Autodesk Inventor part; units mm, degrees
ref_plane "YZ Plane" through (0, 0, 0) normal (1, 0, 0) x (0, 1, 0)
ref_plane "XZ Plane" through (0, 0, 0) normal (0, 1, 0) x (-1, 0, 0)
ref_plane "XY Plane" through (0, 0, 0) normal (0, 0, 1) x (1, 0, 0)
sketch "Sketch1" plane through (0, 0, 0) normal (0, 0, 1) x (1, 0, 0)
  line L0 (75, 0) -> (-75, 0)
  line L1 (-75, 0) -> (-75, 150)
  line L2 (-75, 150) -> (75, 150)
  line L3 (75, 150) -> (75, 0)
  point P0 (0, 0)
  point P1 (0, 0)
  dimension "d1" = 150
  dimension "d2" = 150
extrude "Plate1" add sketch "Sketch1" along normal blind 3
sketch "Sketch2" plane through (0, 0, 0) normal (0, 0, 1) x (1, 0, 0)
  line L0 (-75, 0) -> (-75, 150)
  line L1 (75, 0) -> (-75, 0)
  line L2 (75, 150) -> (75, 0)
  line L3 (-75, 150) -> (75, 150)
  circle A0 centre (0, 75) radius 17.5
  line L4 (45, 40) -> (-45, 40) construction
  line L5 (-45, 40) -> (-45, 110) construction
  line L6 (-45, 110) -> (45, 110) construction
  line L7 (45, 110) -> (45, 40) construction
  line L8 (45, 40) -> (-45, 110) construction
  line L9 (-45, 40) -> (45, 110) construction
  circle A1 centre (-45, 40) radius 4
  circle A2 centre (45, 40) radius 4
  circle A3 centre (45, 110) radius 4
  circle A4 centre (-45, 110) radius 4
  point P0 (0, 0)
  point P1 (0, 0)
  point P2 (75, 75)
  dimension "d3" = 35
  dimension "d4" = 90
  dimension "d5" = 70
  dimension "d7" = 8
extrude "Extrusion1" cut sketch "Sketch2" along normal through all contours A1 | A2 | A3 | A4
sketch "Sketch3" plane through (-72, 150, 3) normal (-1, 0, 0) x (0, -1, 0)
  line L0 (150, 0) -> (0, 0)
  line L1 (0, 0) -> (0, -40)
  line L2 (0, -40) -> (150, -40)
  line L3 (150, -40) -> (150, 0)
edge flange "Flange1" height 40 angle 90 thickness 3 bend radius 3 thickness toward (-1, 0, 0) relief tear relief width 3 relief depth 1.5 corner gap 3 corner form 0 edges at (-75, 75, 0) (75, 75, 0) wall of the first edge with corners at (-72, 0, 3) (-72, 150, 3) (-72, 150, -37) (-72, 0, -37)
bend "Bend1"
corner "Corner1"
sketch "Sketch4" plane through (0, 0, 0) normal (0, 0, 1) x (1, 0, 0)
  circle A0 centre (0, 75) radius 17.5
  line L0 (0, 125) -> (0, 105) construction
  line L1 (-3, 125) -> (-3, 105)
  line L2 (3, 105) -> (3, 125)
  arc A1 (3, 125) -> (-3, 125) centre (0, 125) ccw
  arc A2 (-3, 105) -> (3, 105) centre (0, 105) ccw
  arc A3 (34.641, 95) -> (20, 109.641) centre (0, 75) ccw construction
  arc A4 (37.2391, 96.5) -> (21.5, 112.2391) centre (0, 75) ccw
  arc A5 (32.0429, 93.5) -> (18.5, 107.0429) centre (0, 75) ccw
  arc A6 (32.0429, 93.5) -> (37.2391, 96.5) centre (34.641, 95) ccw
  arc A7 (21.5, 112.2391) -> (18.5, 107.0429) centre (20, 109.641) ccw
  line L3 (0, 75) -> (20, 109.641) construction
  line L4 (0, 75) -> (40, 75) construction
  line L5 (0, 75) -> (34.641, 95) construction
  point P0 (0, 0)
  point P1 (0, 115)
  dimension "d20" = 20
  dimension "d21" = 6
  dimension "d22" = 30
  dimension "d23" = 60
  dimension "d24" = 30
  dimension "d25" = 6
  dimension "d26" = 40
extrude "Extrusion2" [suppressed]
pattern_circular "Circular Pattern1" [suppressed]
equation "\"d1\" = d2"
equation "\"d0\" = Thickness"
equation "\"d10\" = BendReliefWidth"
equation "\"d11\" = BendReliefDepth"
equation "\"d12\" = MinimumRemnant"
equation "\"d13\" = TransitionRadius"
equation "\"d16\" = BendRadius"
equation "\"d17\" = CornerReliefSize"
equation "\"d18\" = GapSize"
equation "\"d19\" = JacobiRadiusSize"
equation "\"BendRadius\" = Thickness"
equation "\"BendReliefWidth\" = Thickness"
equation "\"BendReliefDepth\" = 0.5 * Thickness"
equation "\"CornerReliefSize\" = 4 * Thickness"
equation "\"MinimumRemnant\" = 2 * Thickness"
equation "\"TransitionRadius\" = BendRadius"
equation "\"JacobiRadiusSize\" = BendRadius"
equation "\"GapSize\" = Thickness"
properties part number "FL3.6.2  Motor pillar" material "Stainless Steel"
Could you check a few things on this model? Use its own coordinates, in mm. A direction names the side the tool comes from. Coordinates: 2 decimals unless noted, no trailing zeros. Write each loop counter-clockwise with the first axis right and the second up, starting at its lowest first coordinate (ties: lowest second). Pieces come first, ordered by that corner, then holes. Notation, with made-up numbers: (37.5, 68) - (85.5, 68) arc R23 cw to (85.5, 89) - close; hole circle Ø9 at (49, 60.25). An arc over 180 degrees is marked (long way). Put each result on its own line as item: value. Start each with the question number.
Q1. Thinking about a two-plate mould opening in X: for faces 1 (the flat face through (-1, 76, 0)), 2 (the cylindrical face through (73.289, 73.95, 1.196)), 3 (the flat face through (-23, 150, 1)), which applies, pulls with the +X half, pulls with the -X half, needs draft (parallel to the pull), parting line crosses it, or undercut?
Q2. I'm going to push flat-ended pins straight in: P1, Ø7, axis at x = 45, y = 110, coming from the +Z side; P2, Ø5, axis at x = 32.5, y = 32, coming from the -Z side. Where does each tip first touch, or does it pass through?
Q3. I want a section at C-C on z = -32.5. Write out the boundary of the cut face in (x, y), plus the area to 3 significant figures.
Q4. Please list where these lines run through material, in increasing order: L1, parallel to Y at x = 45, z = 1.1; L2, parallel to X at y = 40, z = 2.2; L3, parallel to X at y = 110, z = -8.
Q5. I want a section at A-A on y = 110. Write out the boundary of the cut face in (x, z).
Q6. Which directions (+Z, -Z, +X, -X, +Y, -Y) give clear straight access to the entire face, cutting with the end or side of a thin tool? Please do faces 4 (the flat face through (-23, 0, 1)), 5 (the flat face through (72, 74, -20)).
Q7. I want a section at B-B on x = 45. Write out the boundary of the cut face in (y, z).
Q8. I want a section at D-D on y = 83.5. Write out the boundary of the cut face in (x, z).
Checks:
1. face 1: undercut
1. face 2: pulls with the +X half
1. face 3: needs draft
2. P1: through
2. P2: z = 0
3. outline: (-75, 0) - (-72, 0) - (-72, 150) - (-75, 150) - close; (72, 0) - (75, 0) - (75, 150) - (72, 150) - close
3. area: 900 mm²
4. L1: 0 to 36, 44 to 106, 114 to 150
4. L2: -71.99 to -49, -41 to 41, 49 to 71.99
4. L3: -75 to -72, 72 to 75
5. outline: (-75, -37) - (-72, -37) - (-72, -3) arc R3 cw to (-69, 0) - (-49, 0) - (-49, 3) - (-69, 3) arc R6 ccw to (-75, -3) - close; (-41, 0) - (41, 0) - (41, 3) - (-41, 3) - close; (49, 0) - (69, 0) arc R3 cw to (72, -3) - (72, -37) - (75, -37) - (75, -3) arc R6 ccw to (69, 3) - (49, 3) - close
6. face 4: +Z, -Z, +X, -X, -Y
6. face 5: -Z, +Y, -Y
7. outline: (0, 0) - (36, 0) - (36, 3) - (0, 3) - close; (44, 0) - (106, 0) - (106, 3) - (44, 3) - close; (114, 0) - (150, 0) - (150, 3) - (114, 3) - close
8. outline: (-75, -37) - (-72, -37) - (-72, -3) arc R3 cw to (-69, 0) - (69, 0) arc R3 cw to (72, -3) - (72, -37) - (75, -37) - (75, -3) arc R6 ccw to (69, 3) - (-69, 3) arc R6 ccw to (-75, -3) - close
